Build history of the part. All positions in model axes, mm. A direction names the side the tool comes from. Round coordinates to 2 decimals unless told otherwise and drop trailing zeros.
from build123d import *

# Parameters (mm, degrees)
SKETCH1_W           = 59
SKETCH1_H           = 49.5
SKETCH1_R           = 3
BOSS_EXTRUDE1_DEPTH = 1.5
BOSS_EXTRUDE2_DEPTH = 49.5
CUT_EXTRUDE1_DEPTH  = 2
CUT_EXTRUDE3_DEPTH  = 65.105869466
CHAMFER3_SIZE       = 2


with BuildPart() as part:
    # Sketch1 → Boss-Extrude1 (new body)
    with BuildSketch(Plane(origin=(0, 0, 0), x_dir=(1, 0, 0), z_dir=(0, 1, 0))):
        Rectangle(SKETCH1_W, SKETCH1_H)
        with Locations(Location((0, 0, 0), (0, 0, 270))):
            Circle(SKETCH1_R, mode=Mode.SUBTRACT)
    extrude(amount=BOSS_EXTRUDE1_DEPTH)

    # Sketch2 → Boss-Extrude2 (add)
    with BuildSketch(Plane(origin=(0, 0, -24.75), x_dir=(-1, 0, 0), z_dir=(0, 0, -1))):
        Polygon((-29.5, 1.5), (29.5, 1.5), (29.5, 2.5), (28.32, 4), (27.14, 2.5), (25.96, 4), (24.78, 2.5), (23.6, 4), (22.42, 2.5), (21.24, 4), (20.06, 2.5), (18.88, 4), (17.7, 2.5), (16.52, 4), (15.34, 2.5), (14.16, 4), (12.98, 2.5), (11.8, 4), (10.62, 2.5), (9.44, 4), (8.26, 2.5), (7.08, 4), (5.9, 2.5), (4.72, 4), (3.54, 2.5), (2.36, 4), (1.18, 2.5), (0, 4), (-1.18, 2.5), (-2.36, 4), (-3.54, 2.5), (-4.72, 4), (-5.9, 2.5), (-7.08, 4), (-8.26, 2.5), (-9.44, 4), (-10.62, 2.5), (-11.8, 4), (-12.98, 2.5), (-14.16, 4), (-15.34, 2.5), (-16.52, 4), (-17.7, 2.5), (-18.88, 4), (-20.06, 2.5), (-21.24, 4), (-22.42, 2.5), (-23.6, 4), (-24.78, 2.5), (-25.96, 4), (-27.14, 2.5), (-28.32, 4), (-29.5, 2.5), align=None)
    extrude(amount=-BOSS_EXTRUDE2_DEPTH)

    # Sketch3 → Cut-Extrude1 (cut)
    with BuildSketch(Plane(origin=(0, 0, 0), x_dir=(-1, 0, 0), z_dir=(0, -1, 0))):
        with BuildLine():
            Line((-1.75, -2.436698586), (-1.75, -5))
            Line((-1.75, -5), (1.75, -5))
            Line((1.75, -5), (1.75, -2.436698586))
            ThreePointArc((1.75, -2.436698586), (0, 3), (-1.75, -2.436698586))
        make_face()
    extrude(amount=-CUT_EXTRUDE1_DEPTH, mode=Mode.SUBTRACT)

    # Sketch4 → Cut-Extrude3 (cut, through all)
    with BuildSketch(Plane(origin=(29.5, 0, 0), x_dir=(0, 0, -1), z_dir=(1, 0, 0))):
        with BuildLine():
            Line((-24, 4), (-24.75, 4))
            Line((-24.75, 4), (-24.75, 3.25))
            ThreePointArc((-24.75, 3.25), (-24.530330086, 3.780330086), (-24, 4))
        make_face()
    cut_extrude3 = extrude(amount=-CUT_EXTRUDE3_DEPTH, mode=Mode.SUBTRACT)

    # Mirror1: Cut-Extrude3 across plane
    add(cut_extrude3.mirror(Plane.XY), mode=Mode.SUBTRACT)

    # Chamfer3
    chamfer3_edges = [part.edges().sort_by_distance(p)[0] for p in [
        (0, 0, 5),
    ]]
    chamfer(chamfer3_edges, length=CHAMFER3_SIZE - 0.0001)  # a hair under: the kernel refuses the full size


solid = part.part
1) Wall check: L1, parallel to X at y = 0.8, z = 0; L2, parallel to X at y = 0.3, z = 3.5; L3, parallel to Z at x = 1, y = 0.5. Give the ranges that are in metal, low to high.
Results:
L1: x = -29.5 to -3, 3 to 29.5
L2: x = -29.5 to -1.75, 1.75 to 29.5
L3: z = -24.75 to -2.83, 6.5 to 24.75
2) Mould opens along Z. For faces 4 (the flat face through (-1.75, 1, 4)), 5 (the flat face through (-6.5, 3.26, -0.35)) say: released by +Z, released by -Z, zero draft, split by the parting line, or undercut.
Results:
face 4: undercut
face 5: zero draft
3) Pin check, flat tip, straight feed: pin 1 Ø12 at (x, z) = (-12, 17.5) entering from +Y. Stop position of the tip, or through.
Results:
pin 1: stops at y = 4
4) Which spindle directions (+Z, -Z, +X, -X, +Y, -Y) get a long thin tool onto all of the face, cutting with end or side? Do faces 1 (the flat face through (-28.92, 3.24, -0.35)), 2 (the flat face through (0, 1, 6)), 3 (the flat face through (-20.66, 3.26, -0.35)). Say none if no direction does.
Results:
face 1: +Z, -Z, -X, +Y
face 2: -Y
face 3: +Z, -Z, +Y
